Source: CAD feature listing. Evaluate the final solid. Frame: model axes, mm. Face numbers are marked on the shaded views. A direction names the side the tool comes from. Give positions to 0.01 mm unless a question says otherwise; leave off trailing zeros. Order: outer loops, then holes, each group sorted by start corner. A loop starts at its lowest first (then second) coordinate and runs counter-clockwise, first axis right, second up. Notation, with made-up numbers: (-22.5, 12) -> (19.5, 12) arc R27 cw to (19.5, 32) -> close; hole circle Ø4 at (41, -14). An arc over 180 degrees is marked (long way). Use CSV: the item, a comma, the result in double quotes.
Autodesk Inventor part; units mm, degrees
ref_plane "Work Plane1" through (2.4384, 14.1421, 14.1421) normal (0, -0.7071, 0.7071) x (1, 0, 0)
ref_plane "YZ Plane" through (0, 0, 0) normal (1, 0, 0) x (0, 1, 0)
ref_plane "XZ Plane" through (0, 0, 0) normal (0, 1, 0) x (-1, 0, 0)
sketch "Sketch1" plane through (0, 0, 0) normal (1, 0, 0) x (0, 1, 0)
  circle A0 centre (0, 0) radius 20
  line L0 (8.5, 8.5) -> (-16.9, 8.5)
  line L1 (8.5, 8.5) -> (8.5, -16.9)
  line L2 (0, 0) -> (0, 20)
  line L3 (0, 20) -> (-60.9241, 20)
  line L4 (-60.9241, 20) -> (-60.9241, 18.5)
  line L5 (-60.9241, 18.5) -> (0, 18.5)
  line L6 (0, 18.5) -> (0, 20)
  line L7 (0, 0) -> (14.1421, 14.1421)
  line L8 (0, 0) -> (20, 0)
  line L9 (-16.9, 8.5) -> (-16.9, 18.5)
  line L10 (-16.9, 8.5) -> (-22.9, 14.5)
  line L11 (-22.9, 14.5) -> (-22.9, 18.5)
  line L12 (12.3744, 12.3744) -> (12.1502, 13.2109)
  line L13 (11.3137, 13.435) -> (9.2071, 11.3284)
  line L14 (9.4313, 10.4919) -> (10.2678, 10.2678)
  line L15 (8.5, 8.5) -> (8.5, -16.9)
  line L16 (20, 0) -> (20, -60.9241)
  line L17 (20, -60.9241) -> (18.5, -60.9241)
  line L18 (18.5, -60.9241) -> (18.5, 0)
  line L19 (8.5, -16.9) -> (18.5, -16.9)
  line L20 (8.5, -16.9) -> (14.5, -22.9)
  line L21 (14.5, -22.9) -> (18.5, -22.9)
  arc A1 (9.2071, 11.3284) -> (9.4313, 10.4919) centre (9.5607, 10.9749) ccw
  arc A2 (12.1502, 13.2109) -> (11.3137, 13.435) centre (11.6673, 13.0815) ccw
  line L22 (10.4311, 10.4311) -> (9.483, 10.6851)
  arc A3 (9.3485, 11.187) -> (9.483, 10.6851) centre (9.5607, 10.9749) ccw
  line L23 (9.3485, 11.187) -> (11.4551, 13.2936)
  arc A4 (11.957, 13.1591) -> (11.4551, 13.2936) centre (11.6673, 13.0815) ccw
  line L24 (11.957, 13.1591) -> (12.2111, 12.2111)
  point P0 (0, 8.5)
  point P1 (-17.7041, 9.3041)
  point P2 (-16.9, 10.6953)
  point P3 (10.6953, -16.9)
  point P4 (9.3041, -17.7041)
  point P5 (18.5, 0)
  dimension "d0" = 40
  dimension "d1" = 25.4
  dimension "d2" = 1.5
  dimension "d4" = 45
  dimension "d6" = 45
  dimension "d7" = 4
  dimension "d8" = 10
  dimension "d10" = 2.5
  dimension "d11" = 2.5
  dimension "d12" = 60
  dimension "d13" = 1.5
  dimension "d15" = 0.5
  dimension "d16" = 0.2
extrude "Extrusion1" add sketch "Sketch1" along normal blind 61 contours L8 L1 L7 A0 | L18 L19 A0 | A0 L19 L1 L8 L18 | L19 L18 L21 L20 A0 | A0 L20 L19
sketch "Sketch3" plane through (0, 18.5, 0) normal (0, 1, 0) x (1, 0, 0)
  line L0 (0, 22.9) -> (0, 0)
  line L1 (0, 0) -> (61, 0)
  line L2 (61, 22.9) -> (61, 0)
  line L3 (0, 22.9) -> (61, 22.9)
  line L4 (0, 16.9) -> (61, 16.9)
  line L5 (13.3257, 4) -> (11.6514, 6.9)
  line L6 (11.6514, 6.9) -> (13.3257, 9.8)
  line L7 (13.3257, 9.8) -> (16.6743, 9.8)
  line L8 (16.6743, 9.8) -> (18.3486, 6.9)
  line L9 (18.3486, 6.9) -> (16.6743, 4)
  line L10 (16.6743, 4) -> (13.3257, 4)
  circle A0 centre (15, 6.9) radius 1.65
  point P0 (0, 0)
  dimension "d28" = 5.8
  dimension "d29" = 10
  dimension "d30" = 15
  dimension "d31" = 3.3
extrude "Extrusion4" cut sketch "Sketch3" against normal blind 6 contours L5 L6 L7 L8 L9 L10 | A0
extrude "Extrusion5" cut sketch "Sketch3" against normal through all contours A0
sketch "Sketch4" plane through (0, 14.5, -22.9) normal (0, 0, -1) x (-1, 0, 0)
  line L0 (0, -6) -> (0, 0)
  line L1 (0, 0) -> (0, 4)
  line L2 (0, 4) -> (0, 5.5)
  line L3 (0, -6) -> (-61, -6)
  line L4 (0, 5.5) -> (-61, 5.5)
  line L5 (0, 5.5) -> (-4.787, -6)
  point P0 (0, -14.5)
  dimension "d36" = 112.6
ref_plane "Work Plane1" through (2.4384, 14.1421, 14.1421) normal (0, -0.7071, 0.7071) x (1, 0, 0)
sketch "Sketch5" plane through (2.4384, 14.1421, 14.1421) normal (0, -0.7071, 0.7071) x (1, 0, 0)
  circle A0 centre (12.5616, -3.9896) radius 1.5
  line L0 (-2.4384, 0) -> (-2.4384, -7.9792)
  line L1 (-2.4384, -7.9792) -> (58.5616, -7.9792)
  line L2 (58.5616, 0) -> (58.5616, -7.9792)
  line L3 (-2.4384, 0) -> (58.5616, 0)
  point P0 (-2.4384, -3.9896)
  dimension "d42" = 3
  dimension "d55" = 15
extrude "Extrusion7" cut sketch "Sketch5" against normal blind 3 contours A0
ref_plane "Work Plane2" through (30.5, 0, 0) normal (-1, 0, 0) x (0, 0, 1)
mirror "Mirror1" about plane through (30.5, 0, 0) normal (-1, 0, 0) of "Extrusion7", "Extrusion5", "Extrusion4"
properties part number "ESQUINA_REDONDEADA_R20" material "Steel, Mild, Welded"
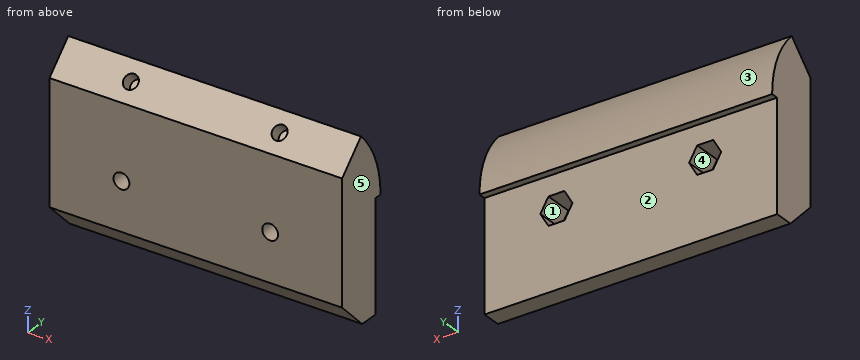
1. Mould query, pull axis Z, two halves, no side actions, for the marked faces 1, 2 and 3. Classes: released by +Z, released by -Z, zero draft, split by the parting line, or undercut.
Answer below:
face 1,"undercut"
face 2,"zero draft"
face 3,"released by +Z"
2. Pin query (flat end, axial travel): P1, Ø0.8, axis at x = 26, y = 19, coming from the -Z side; P2, Ø8, axis at x = 8, z = -19, coming from the +Y side; P3, Ø6, axis at x = 34.5, y = 11, coming from the +Z side; P4, Ø2, axis at x = 46, z = -6.9, coming from the -Y side. Return the tip coordinate at first contact, or that it passes through.
Answer below:
P1,"stops at z = 0"
P2,"stops at y = 18.5"
P3,"stops at z = 14"
P4,"passes through"
3. Access query for the marked faces 4 and 5. Directions: +Z, -Z, +X, -X, +Y, -Y. A direction counts if a zero-diameter tool reaches every point of the face in a straight line with its end or side. Return the directions, or none.
Answer below:
face 4,"+Y"
face 5,"+Z, -Z, +X, +Y, -Y"
4. Section query A-A on x = 15. Return loops of the section in (y, z).
Answer below:
outline,"(8.5, -16.9) -> (14.5, -22.9) -> (18.5, -22.9) -> (18.5, -9.8) -> (12.5, -9.8) -> (12.5, -8.55) -> (8.5, -8.55) -> close; (8.5, -5.25) -> (12.5, -5.25) -> (12.5, -4) -> (18.5, -4) -> (18.5, 0) -> (20, 0) arc R20 ccw to (14.14, 14.14) -> (12.38, 12.38) -> (14.5, 10.26) -> (12.38, 8.14) -> (10.26, 10.26) -> (8.5, 8.5) -> close"
5. Section query B-B on x = 39. Return loops of the section in (y, z).
Answer below:
outline,"(8.5, -16.9) -> (14.5, -22.9) -> (18.5, -22.9) -> (18.5, 0) -> (20, 0) arc R20 ccw to (14.14, 14.14) -> (8.5, 8.5) -> close"
6. Section query C-C on y = 17. Return loops of the section in (x, z), plus the area to 3 significant figures.
Answer below:
outline,"(0, -22.9) -> (61, -22.9) -> (61, 10.54) -> (0, 10.54) -> close; hole (11.65, -6.9) -> (13.33, -9.8) -> (16.67, -9.8) -> (18.35, -6.9) -> (16.67, -4) -> (13.33, -4) -> close; hole (42.65, -6.9) -> (44.33, -9.8) -> (47.67, -9.8) -> (49.35, -6.9) -> (47.67, -4) -> (44.33, -4) -> close"
area,"1,980 mm²"
7. Ray query, line 1 along X through (y, z) = (17.75, -6.5); line 2 along Z through (x, y) = (46, 10.35); line 3 along Z through (x, y) = (46, 10.2). Return the intervals inside material, ascending.
Answer below:
line 1,"x = 0 to 11.88, 18.12 to 42.88, 49.12 to 61"
line 2,"z = -18.75 to -8.55, -5.25 to 10.17"
line 3,"z = -18.6 to -8.55, -5.25 to 10.2"
